from build123d import *

# Parameters (mm, degrees)
SKETCH2_W          = 10
SKETCH2_H          = 6
SKETCH2_W_2        = 6
SKETCH2_H_2        = 4
SKETCH3_R          = 3
CUT_EXTRUDE1_DEPTH = 140.45967159


with BuildPart() as part:
    # Sketch2 → Revolve1 (revolve)
    with BuildSketch(Plane.XY, mode=Mode.PRIVATE) as revolve1_sk:
        Polygon((22, 6), (22, 0), (104, 0), (104, 6), (104, 8), (22, 8), align=None)
        with Locations((109, 3)):
            Rectangle(SKETCH2_W, SKETCH2_H)
        with BuildLine():
            Line((114, 6), (114, 0))
            Line((114, 0), (123, 0))
            ThreePointArc((123, 0), (126, 3), (129, 0))
            Line((129, 0), (138, 0))
            Line((138, 0), (138, 9))
            Line((138, 9), (114, 9))
            Line((114, 9), (114, 6))
        make_face()
        Polygon((13, 4), (13, 0), (22, 0), (22, 6), (13, 6), align=None)
        Polygon((0, 6), (0, 0), (7, 0), (7, 4), (7, 6), align=None)
        with Locations((10, 2)):
            Rectangle(SKETCH2_W_2, SKETCH2_H_2)
    revolve(revolve1_sk.sketch.rotate(Axis((-35.742937112, 0, 0), (1, 0, 0)), 90), axis=Axis((-35.742937112, 0, 0), (1, 0, 0)))

    # Sketch3 → Cut-Extrude1 (cut, through all)
    with BuildSketch(Plane.XY.offset(9)):
        with Locations((127.319310505, 0)):
            Circle(SKETCH3_R)
    extrude(amount=-CUT_EXTRUDE1_DEPTH, mode=Mode.SUBTRACT)


solid = part.part
Can you work these out from the model? Positions are in its coordinate system, mm. A direction names the side the tool comes from. Give positions to 0.01 mm unless a question says otherwise; leave off trailing zeros. Order: outer loops, then holes, each group sorted by start corner. A loop starts at its lowest first (then second) coordinate and runs counter-clockwise, first axis right, second up. Notation, with made-up numbers: M 23,49 L 37,49 A33 ccw 37,83 Z; hole C 30.5,55.5 d8. An arc over 180 degrees is marked long. Use one line per item in the form item = value. Start each with the question number.
Item 1: Will these pins go through, and if not, where does the flat tip stop? pin 1 Ø3 at (x, z) = (35.5, -5.5) entering from -Y; pin 2 Ø1.5 at (x, z) = (61, 2) entering from +Y; pin 3 Ø10 at (x, y) = (69.5, 3) entering from +Z.
Item 2: If we section it at C-C (x = 44): Write out the boundary of the cut face in (y, z).
Item 3: We'd pull the mould along Y, two halves only. Please class faces 4 (the cylindrical face through (109.07, -1.802, 5.723)), 5 (the flat face through (138, 0, 0)), 6 (the cylindrical face through (130.18, 0.9, 0.12)): +Y half, -Y half, draft (parallel to the pull), parting line (faces both ways), or undercut.
Item 4: If we section it at B-B (z = 0): Write out the boundary of the cut face in (x, y).
Item 5: For faces 1 (the flat face through (0, 0, 0)), 2 (the cylindrical face through (17.437, -1.802, 5.723)), 3 (the flat face through (13, 3.92, -1.42)), which set-ups out of +Z, -Z, +X, -X, +Y, -Y let a thin tool reach every point of the face, with its end or its side?
Item 6: If I drill on line 1 along X through (y, z) = (-3.5, 6.5); line 2 along X through (y, z) = (-1, -7); line 3 along X through (y, z) = (-1.25, 7.25), over which ranges is the centre line in solid material (lowest first)?
Outcome:
q1.pin_1 = -6.93
q1.pin_2 = 7.9
q1.pin_3 = 8
q2.outline = C 0,0 d16
q3.face_4 = parting line
q3.face_5 = draft
q3.face_6 = undercut
q4.outline = M 0,-6 L 7,-6 L 7,-4 L 13,-4 L 13,-6 L 22,-6 L 22,-8 L 104,-8 L 104,-6 L 114,-6 L 114,-9 L 138,-9 L 138,9 L 114,9 L 114,6 L 104,6 L 104,8 L 22,8 L 22,6 L 13,6 L 13,4 L 7,4 L 7,6 L 0,6 Z; hole M 126.66,-2.93 A3 ccw long 126.66,2.93 A3 ccw long Z
q5.face_1 = +Z, -Z, -X, +Y, -Y
q5.face_2 = -X
q5.face_3 = none
q6.line_1 = 22 to 104, 114 to 138
q6.line_2 = 22 to 104, 114 to 124.49, 130.15 to 138
q6.line_3 = 22 to 104, 114 to 124.59, 130.05 to 138
